Design review of the part shown in the three views and the two pictorial views. Dimensions are in mm from the part's minimum x, y and z. Round coordinates to 2 decimals unless told otherwise and drop trailing zeros. Loops run counter-clockwise (first coordinate to the right, second up) from the corner with the lowest first, then second, coordinate; pieces in that order, holes last. Notation, with made-up numbers: (67, -12) - (94, -12) arc R20 ccw to (94, 12) - close; hole circle Ø4 at (64, 16). An arc over 180 degrees is marked (long way). Return JSON: item names as keys, results as strings. Group by question number.
(1) Clearance check with flat-ended pins moving along their axes: pin 1 (1.5 mm diameter, centred on y = 14, z = 9, fed in from -X); pin 2 (3 mm diameter, centred on x = 105.5, y = 108, fed in from +Z) (3 decimals); pin 3 (6 mm diameter, centred on y = 19, z = 5.5, fed in from +X). State where each tip first meets the part, or that it passes through.
(2) We need section D-D, the plane y = 10. Write out the cut boundary in (x, z), and give its area (3 significant figures).
(3) Wall thickness on L1, parallel to X at y = 106, z = 13.5; L2, parallel to Z at x = 30, y = 104.5 (1 decimal); L3, parallel to Y at x = 103, z = 15.25: over which ranges is each line inside the solid? List them lowest first. Write a range as [from, to].
(4) We need section B-B, the plane z = 7. Write out the cut boundary in (x, y), and give its area (3 significant figures).
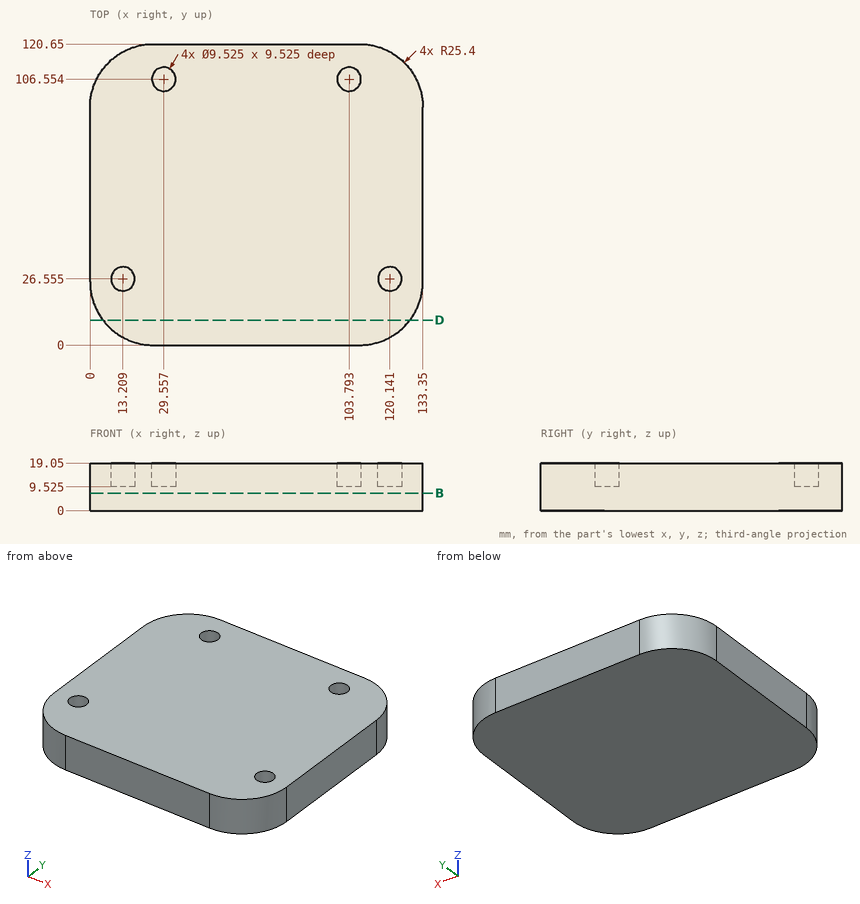
Solutions:
{
 "1": {"pin 1": "x = 2.34", "pin 2": "z = 9.525", "pin 3": "x = 133.12"},
 "2": {"outline": "(5.2, 0) - (128.15, 0) - (128.15, 19.05) - (5.2, 19.05) - close", "area": "2,340 mm^2"},
 "3": {"L1": "[2.39, 24.83], [34.29, 99.06], [108.52, 130.96]", "L2": "[0, 9.5]", "L3": "[0, 101.86], [111.25, 120.65]"},
 "4": {"outline": "(0, 25.4) arc R25.4 ccw to (25.4, 0) - (107.95, 0) arc R25.4 ccw to (133.35, 25.4) - (133.35, 95.25) arc R25.4 ccw to (107.95, 120.65) - (25.4, 120.65) arc R25.4 ccw to (0, 95.25) - close", "area": "15,500 mm^2"}
}
